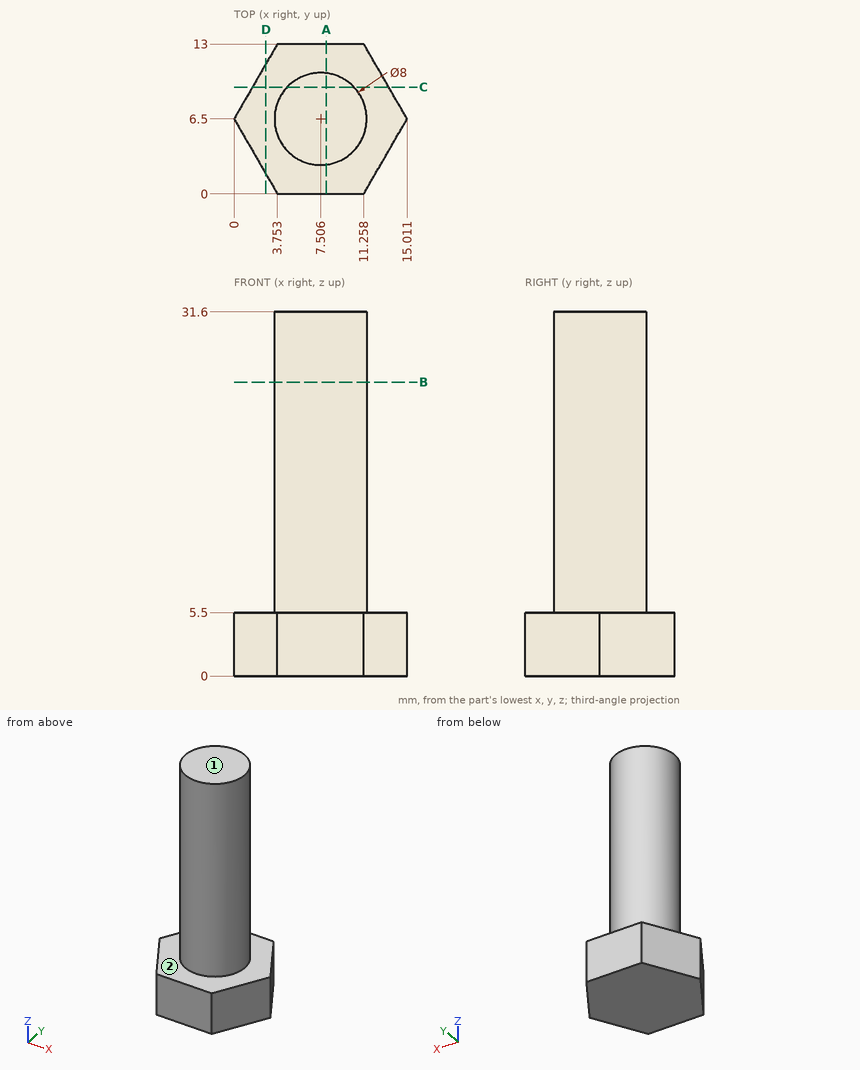
Geometry: see drawing. Coordinates: mm, zero at the bounding-box minimum. A direction names the side the tool comes from. Round coordinates to 2 decimals unless told otherwise and drop trailing zeros. Loops run counter-clockwise (first coordinate to the right, second up) from the corner with the lowest first, then second, coordinate; pieces in that order, holes last. Notation, with made-up numbers: M 85,-12.75 L 97,-12.75 A26 cw 97,5.25 Z; hole C 30.25,-38.75 d1. An arc over 180 degrees is marked long. Use a Markdown table: item, result. Add a question column.
1. Cut plane D-D, the plane x = 2.75. Output: boundary loops of the cut face in (y, z), and give its area (3 significant figures).
2. Cut plane C-C, the plane y = 9.25. Output: boundary loops of the cut face in (x, z).
3. Ray query, line 1 along Z through (x, y) = (2, 8); line 2 along X through (y, z) = (6.75, 8.5); line 3 along X through (y, z) = (8.5, 2) (1 decimal). Return the intervals inside material, ascending. Write a range as [from, to].
4. Cut plane A-A, the plane x = 8. Output: boundary loops of the cut face in (y, z).
5. Cut plane B-B, the plane z = 25.5. Output: boundary loops of the cut face in (x, y) (1 decimal).
6. Contact query for flat-ended pins moving along their axis: pin 1 (2 mm diameter, centred on x = 5.5, z = 25, fed in from +Y); pin 2 (3 mm diameter, centred on y = 4, z = 22.5, fed in from +X); pin 3 (6 mm diameter, centred on y = 8.5, z = 15.5, fed in from +X); pin 4 (1.5 mm diameter, centred on x = 11, y = 7.5, fed in from -Z). Output: stop coordinate, or through.
7. Set-up query: the marked faces 1 and 2. Return all of +Z, -Z, +X, -X, +Y, -Y with unobstructed straight access to the full face (end or side cutting, diameter ignored); none if empty.
Solution:
| question | item | result |
|---|---|---|
| 1 | outline | M 1.74,0 L 11.26,0 L 11.26,5.5 L 1.74,5.5 Z |
| 1 | area | 52.4 mm2 |
| 2 | outline | M 1.59,0 L 13.42,0 L 13.42,5.5 L 10.41,5.5 L 10.41,31.6 L 4.6,31.6 L 4.6,5.5 L 1.59,5.5 Z |
| 3 | line 1 | z = [0, 5.5] |
| 3 | line 2 | x = [3.51, 11.5] |
| 3 | line 3 | x = [1.2, 13.9] |
| 4 | outline | M 0,0 L 13,0 L 13,5.5 L 10.47,5.5 L 10.47,31.6 L 2.53,31.6 L 2.53,5.5 L 0,5.5 Z |
| 5 | outline | C 7.5,6.5 d8 |
| 6 | pin 1 | stops at y = 10.37 |
| 6 | pin 2 | stops at x = 11.38 |
| 6 | pin 3 | stops at x = 11.51 |
| 6 | pin 4 | stops at z = 0 |
| 7 | face 1 | +Z, +X, -X, +Y, -Y |
| 7 | face 2 | +Z |
